Part model, mm, in its own coordinate system. A direction names the side the tool comes from. Give positions to 0.01 mm unless a question says otherwise; leave off trailing zeros. Write each loop counter-clockwise with the first axis right and the second up, starting at its lowest first coordinate (ties: lowest second). Pieces come first, ordered by that corner, then holes. Notation, with made-up numbers: M 13,-20.75 L 61,-20.75 A18 ccw 61,1.25 Z; hole C 79.5,49 d6. An arc over 180 degrees is marked long. Use a Markdown table: item, result. Add a question column.
from build123d import *

# Parameters (mm, degrees)
SKETCH_1_R          = 8.5
EXTRUDE_1_DEPTH     = 22
SKETCH_2_R          = 11.5
EXTRUDE_2_DEPTH     = 30
SKETCH_3_R          = 8.5
EXTRUDE_3_DEPTH     = 48
CUT_EXTRUDE_START   = -5.5
CUT_EXTRUDE_1_DEPTH = 48
CUT_EXTRUDE_2_DEPTH = 5.5
M8X1_0_1_D          = 7
M8X1_0_1_DEPTH      = 18
M8X1_0_1_TIP        = 2.103012167


with BuildPart() as part:
    # 草图1 → 凸台-拉伸1 (new body)
    with BuildSketch(Plane(origin=(0, 0, 0), x_dir=(1, 0, 0), z_dir=(0, 1, 0))):
        with Locations(Location((0, 0, 0), (0, 0, 270))):
            Circle(SKETCH_1_R)
    extrude(amount=EXTRUDE_1_DEPTH)

    # 草图2 → 凸台-拉伸2 (add)
    with BuildSketch(Plane(origin=(0, 22, 0), x_dir=(1, 0, 0), z_dir=(0, 1, 0))):
        with Locations(Location((0, 0, 0), (0, 0, 270))):
            Circle(SKETCH_2_R)
    extrude(amount=EXTRUDE_2_DEPTH)

    # 草图3 → 凸台-拉伸3 (add)
    with BuildSketch(Plane(origin=(0, 52, 0), x_dir=(1, 0, 0), z_dir=(0, 1, 0))):
        with Locations(Location((0, 0, 0), (0, 0, 270))):
            Circle(SKETCH_3_R)
    extrude(amount=EXTRUDE_3_DEPTH)

    # 草图4 → 切除-拉伸1 (cut)
    with BuildSketch(Plane(origin=(0, 0, 0), x_dir=(0, 0, -1), z_dir=(1, 0, 0)).offset(CUT_EXTRUDE_START)):
        with BuildLine():
            Line((2.5, 17.5), (2.5, 4.5))
            ThreePointArc((2.5, 4.5), (0, 2), (-2.5, 4.5))
            Line((-2.5, 4.5), (-2.5, 17.5))
            ThreePointArc((-2.5, 17.5), (0, 20), (2.5, 17.5))
        make_face()
    extrude(amount=-CUT_EXTRUDE_1_DEPTH, mode=Mode.SUBTRACT)

    # 草图5 → 切除-拉伸2 (cut)
    with BuildSketch(Plane(origin=(0, 0, 0), x_dir=(0, 0, -1), z_dir=(1, 0, 0)).offset(CUT_EXTRUDE_START)):
        with BuildLine():
            Line((2.5, 96), (2.5, 87.133575026))
            ThreePointArc((2.5, 87.133575026), (0, 84.633575026), (-2.5, 87.133575026))
            Line((-2.5, 87.133575026), (-2.5, 96))
            ThreePointArc((-2.5, 96), (0, 98.5), (2.5, 96))
        make_face()
    extrude(amount=-CUT_EXTRUDE_2_DEPTH, mode=Mode.SUBTRACT)

    # M8x1.0 螺纹孔1
    with Locations(Plane(origin=(0, 100, 0), x_dir=(1, 0, 0), z_dir=(0, 1, 0))):
        with Locations((0, 0)):
            Hole(M8X1_0_1_D / 2, depth=M8X1_0_1_DEPTH)
            with Locations((0, 0, -(M8X1_0_1_DEPTH + M8X1_0_1_TIP / 2))):  # 118° drill point
                Cone(0, M8X1_0_1_D / 2, M8X1_0_1_TIP, mode=Mode.SUBTRACT)


solid = part.part
1. Cut at D-D (y = 56). Write the cut outline in (x, z).
2. Cut at A-A (z = -5.5). Write the cut outline in (x, y), then the cut area to 3 significant figures.
3. Tool access for faces 1 (the flat face through (0, 100, 4)), 2 (the cylindrical face through (8.428, 75.664, -1.107)), 3 (the cylindrical face through (9.7, 36.79, 6.18)), 4 (the flat face through (-8, 22, -4)), 5 (the flat face through (-7, 92, 2.5)): list every direction of +Z, -Z, +X, -X, +Y, -Y with a clear straight run to the whole face (end or side of a thin tool).
4. Mould opens along Y. For faces 6 (the flat face through (-8, 52, -4)), 7 (the cylindrical face through (-3.233, 90.874, 1.341)), 8 (the flat face through (-7, 11, -2.5)), 9 (the flat face through (0, 0, 0)) say: released by +Y, released by -Y, zero draft, split by the parting line, or undercut.
5. Cut at C-C (x = 6.5). Write the cut outline in (y, z).
6. Drill centre lines: probe 1 along Y at (x, z) = (-5.5, -7.5); probe 2 along X at (y, z) = (30, 0.25); probe 3 along X at (y, z) = (75, -0.5). Where is each one in solid material? Low to high. Write a range as [from, to].
7. Flat gauge pins, fed straight in: pin 1 (5.5 mm diameter, centred on y = 90, z = 0, fed in from -X); pin 2 (1.5 mm diameter, centred on x = -4.5, y = 88, fed in from +Z); pin 3 (2 mm diameter, centred on y = 74, z = -3, fed in from -X); pin 4 (11 mm diameter, centred on x = 0, z = 0, fed in from -Y). Where does each tip first touch, or does it go through?
8. Cut at B-B (y = 37). Write the cut outline in (x, z).
A:
| question | item | result |
|---|---|---|
| 1 | outline | C 0,0 d17 |
| 2 | outline | M -10.1,22 L -6.48,22 L -6.48,0 L 6.48,0 L 6.48,22 L 10.1,22 L 10.1,52 L 6.48,52 L 6.48,100 L -6.48,100 L -6.48,52 L -10.1,52 Z |
| 2 | area | 1,510 mm² |
| 3 | face 1 | +Z, -Z, +X, -X, +Y |
| 3 | face 2 | +Y |
| 3 | face 3 | +Y, -Y |
| 3 | face 4 | -Y |
| 3 | face 5 | -X |
| 4 | face 6 | released by +Y |
| 4 | face 7 | zero draft |
| 4 | face 8 | undercut |
| 4 | face 9 | released by -Y |
| 5 | outline | M 0,-5.48 L 22,-5.48 L 22,-9.49 L 52,-9.49 L 52,-5.48 L 100,-5.48 L 100,5.48 L 52,5.48 L 52,9.49 L 22,9.49 L 22,5.48 L 0,5.48 Z |
| 6 | probe 1 | y = [22, 52] |
| 6 | probe 2 | x = [-11.5, 11.5] |
| 6 | probe 3 | x = [-8.49, 8.49] |
| 7 | pin 1 | stops at x = -8.12 |
| 7 | pin 2 | stops at z = 7.63 |
| 7 | pin 3 | stops at x = -8.26 |
| 7 | pin 4 | stops at y = 0 |
| 8 | outline | C 0,0 d23 |
